Geometry: final body of the model. Coordinates: model frame, mm. A direction names the side the tool comes from. Coordinates: 2 decimals unless noted, no trailing zeros. Order: outer loops, then holes, each group sorted by start corner. A loop starts at its lowest first (then second) coordinate and runs counter-clockwise, first axis right, second up. Notation, with made-up numbers: M 41,53 L 59,53 A6 ccw 59,62 Z; hole C 39,-13 d6. An arc over 180 degrees is marked long. Use CSV: the item, a comma, the result in double quotes. Start each with the question number.
1. Section query B-B on y = 8.75. Return the cut outline in (x, z).
2. First-contact query: P1, Ø5, axis at x = 6.5, z = 18, coming from the +Y side; P2, Ø1.8, axis at x = 0, z = 0, coming from the -Y side; P3, Ø1, axis at y = 1.5, z = -18.5, coming from the -X side; P4, Ø3, axis at x = 16.5, y = 4.5, coming from the +Z side. Flat tips, straight axial feed; report the tip coordinate or a pass-through.
3. Section query A-A on z = 0. Return the cut outline in (x, y).
4. Section query D-D on z = 21. Return the cut outline in (x, y).
5. Pull-direction query (Z, two-part tool) for faces 3 (the flat face through (-7, 0, 0)), 4 (the cylindrical face through (-21, 5, -28)), 5 (the cylindrical face through (0.33, 7.465, -7.493)); classes: pulls with the +Z half, pulls with the -Z half, needs draft (parallel to the pull), parting line crosses it, or undercut.
6. Set-up query: faces 1 (the cylindrical face through (0.45, 0.51, 1.43)), 2 (the cylindrical face through (-2.55, 5.44, 0.02)). Return all of +Z, -Z, +X, -X, +Y, -Y with unobstructed straight access to the full face (end or side cutting, diameter ignored); none if empty.
7. Section query C-C on y = 3.75. Return the cut outline in (x, z), and give its area (3 significant figures).
8. Material intervals for line 1 (X direction, y = 5.5, z = 4); line 2 (X direction, y = 5.5, z = 3.5); line 3 (X direction, y = 0.85, z = 0), sorted ascending.
from build123d import *

# Parameters (mm, degrees)
IZIM1_R                     = 35
Y_KSEKLIK_EKSTR_ZYON1_DEPTH = 5
IZIM2_R                     = 7.5
Y_KSEKLIK_EKSTR_ZYON2_DEPTH = 5
KES_EKSTR_ZYON1_START       = -4
KES_EKSTR_ZYON1_DEPTH       = 4
IZIM4_R                     = 1.5
KES_EKSTR_ZYON2_DEPTH       = 4
IZIM5_R                     = 35
IZIM5_R_2                   = 30
Y_KSEKLIK_EKSTR_ZYON3_DEPTH = 5


with BuildPart() as part:
    # Çizim1 → Yükseklik-Ekstrüzyon1 (new body)
    with BuildSketch(Plane(origin=(0, 0, 0), x_dir=(1, 0, 0), z_dir=(0, 1, 0))):
        with Locations(Location((0, 0, 0), (0, 0, 270))):
            Circle(IZIM1_R)
    extrude(amount=Y_KSEKLIK_EKSTR_ZYON1_DEPTH)

    # Çizim2 → Yükseklik-Ekstrüzyon2 (add)
    with BuildSketch(Plane(origin=(0, 5, 0), x_dir=(1, 0, 0), z_dir=(0, 1, 0))):
        with Locations(Location((0, 0, 0), (0, 0, 270))):
            Circle(IZIM2_R)
        with BuildLine():
            Line((-2.062159063, 1.5), (2.062159063, 1.5))
            ThreePointArc((2.062159063, 1.5), (2.55, 0), (2.062159063, -1.5))
            Line((2.062159063, -1.5), (-2.062159063, -1.5))
            ThreePointArc((-2.062159063, -1.5), (-2.55, 0), (-2.062159063, 1.5))
        make_face(mode=Mode.SUBTRACT)
    extrude(amount=Y_KSEKLIK_EKSTR_ZYON2_DEPTH)

    # Çizim3 → Kes-Ekstrüzyon1 (cut)
    with BuildSketch(Plane(origin=(0, 5, 0), x_dir=(1, 0, 0), z_dir=(0, 1, 0)).offset(KES_EKSTR_ZYON1_START)):
        with BuildLine():
            Line((-2.062159063, 1.5), (2.062159063, 1.5))
            ThreePointArc((2.062159063, 1.5), (2.55, 0), (2.062159063, -1.5))
            Line((2.062159063, -1.5), (-2.062159063, -1.5))
            ThreePointArc((-2.062159063, -1.5), (-2.55, 0), (-2.062159063, 1.5))
        make_face()
    extrude(amount=KES_EKSTR_ZYON1_DEPTH, mode=Mode.SUBTRACT)

    # Çizim4 → Kes-Ekstrüzyon2 (cut)
    with BuildSketch(Plane(origin=(0, 1, 0), x_dir=(1, 0, 0), z_dir=(0, 1, 0))):
        with Locations(Location((0, 0, 0), (0, 0, 270))):
            Circle(IZIM4_R)
    extrude(amount=-KES_EKSTR_ZYON2_DEPTH, mode=Mode.SUBTRACT)

    # Çizim5 → Yükseklik-Ekstrüzyon3 (add)
    with BuildSketch(Plane(origin=(0, 5, 0), x_dir=(1, 0, 0), z_dir=(0, 1, 0))):
        with Locations(Location((0, 0, 0), (0, 0, 270))):
            Circle(IZIM5_R)
        with Locations(Location((0, 0, 0), (0, 0, 270))):
            Circle(IZIM5_R_2, mode=Mode.SUBTRACT)
    extrude(amount=Y_KSEKLIK_EKSTR_ZYON3_DEPTH)


solid = part.part
Results list:
1,outline,"C 0,0 d70; C 0,0 d15; hole C 0,0 d60; hole M -2.06,-1.5 L 2.06,-1.5 A2.55 ccw 2.06,1.5 L -2.06,1.5 A2.55 ccw Z"
2,P1,"stops at y = 5"
2,P2,"passes through"
2,P3,"stops at x = -30.02"
2,P4,"stops at z = 31.62"
3,outline,"M -35,0 L -1.5,0 L -1.5,1 L -2.55,1 L -2.55,10 L -7.5,10 L -7.5,5 L -30,5 L -30,10 L -35,10 Z; M 1.5,0 L 35,0 L 35,10 L 30,10 L 30,5 L 7.5,5 L 7.5,10 L 2.55,10 L 2.55,1 L 1.5,1 Z"
4,outline,"M -28,0 L 28,0 L 28,10 L 21.42,10 L 21.42,5 L -21.42,5 L -21.42,10 L -28,10 Z"
5,face 3,"needs draft"
5,face 4,"parting line crosses it"
5,face 5,"undercut"
6,face 1,"+Y, -Y"
6,face 2,"+Y"
7,outline,"C 0,0 d70; hole M -2.06,-1.5 L 2.06,-1.5 A2.55 ccw 2.06,1.5 L -2.06,1.5 A2.55 ccw Z"
7,area,"3,830 mm²"
8,line 1,"x = -34.77 to -29.73, -6.34 to 6.34, 29.73 to 34.77"
8,line 2,"x = -34.82 to -29.8, -6.63 to 6.63, 29.8 to 34.82"
8,line 3,"x = -35 to -1.5, 1.5 to 35"
